Can you work these out from the model? Positions are in its coordinate system, mm. A direction names the side the tool comes from. Coordinates: 2 decimals unless noted, no trailing zeros. Loops run counter-clockwise (first coordinate to the right, second up) from the corner with the lowest first, then second, coordinate; pieces in that order, holes last.
Autodesk Inventor part; units mm, degrees
ref_plane "YZ Plane" through (0, 0, 0) normal (1, 0, 0) x (0, 1, 0)
ref_plane "XZ Plane" through (0, 0, 0) normal (0, 1, 0) x (-1, 0, 0)
ref_plane "XY Plane" through (0, 0, 0) normal (0, 0, 1) x (1, 0, 0)
sketch "Sketch1" plane through (0, 0, 0) normal (0, 1, 0) x (-1, 0, 0)
  line L0 (0, 0) -> (33, 0)
  line L1 (33, 0) -> (33, -12)
  line L2 (33, -12) -> (0, -12)
  line L3 (0, -12) -> (0, 0)
  circle A0 centre (26, -6) radius 3.25
  circle A1 centre (7, -6) radius 3.25
  dimension "d0" = 12
  dimension "d1" = 33
  dimension "d2" = 6.5
  dimension "d3" = 6.5
  dimension "d4" = 7
  dimension "d6" = 6
  dimension "d7" = 6
  dimension "d9" = 19
extrude "Extrusion1" add sketch "Sketch1" along normal mid plane 14
sketch "Sketch2" plane through (0, -7, -12) normal (0, 0, -1) x (-1, 0, 0)
  circle A0 centre (16.5, 7) radius 3.1
  line L0 (33, 14) -> (33, 0)
  line L1 (33, 0) -> (0, 0)
  point P0 (0, 7)
  dimension "d12" = 6.2
  dimension "d14" = 16.5
  dimension "d20" = 7
extrude "Extrusion2" cut sketch "Sketch2" against normal up to next
sketch "Sketch3" plane through (-33, -7, 0) normal (0, 0, 1) x (1, 0, 0)
  circle A0 centre (16.5, 7) radius 3.1
  line L0 (16.5, 13.0044) -> (21.7, 10.0022)
  line L1 (21.7, 10.0022) -> (21.7, 3.9978)
  line L2 (21.7, 3.9978) -> (16.5, 0.9956)
  line L3 (16.5, 0.9956) -> (11.3, 3.9978)
  line L4 (11.3, 3.9978) -> (11.3, 10.0022)
  line L5 (11.3, 10.0022) -> (16.5, 13.0044)
  line L6 (0, 14) -> (33, 14)
  line L7 (0, 14) -> (0, 0)
  point P0 (33, 7)
  dimension "d17" = 5.2
extrude "Extrusion3" cut sketch "Sketch3" against normal blind 5
properties part number "smallSprocketFixture" material "ABS Plastic"
Item 1: Suppose I cut it at C-C, the plane x = -26. Please give me the cut outline in (y, z).
Results are:
outline: (-7, -12) - (7, -12) - (7, -9.25) - (-7, -9.25) - close; (-7, -2.75) - (7, -2.75) - (7, 0) - (-7, 0) - close
Item 2: Suppose I cut it at B-B, the plane y = 0. Please give me the cut outline in (x, z).
Results are:
outline: (-33, -12) - (-19.6, -12) - (-19.6, -5) - (-21.7, -5) - (-21.7, 0) - (-33, 0) - close; (-13.4, -12) - (0, -12) - (0, 0) - (-11.3, 0) - (-11.3, -5) - (-13.4, -5) - close; hole circle Ø6.5 at (-26, -6); hole circle Ø6.5 at (-7, -6)
Item 3: I need wall thicknesses on line 1 along Z through (x, y) = (-26, 0); line 2 along Y through (x, z) = (-16.5, -7); line 3 along X through (y, z) = (0.25, -6.75). Which ranges of each line are inside material? Lowest first, please.
Results are:
line 1: z = -12 to -9.25, -2.75 to 0
line 2: y = -7 to -3.1, 3.1 to 7
line 3: x = -33 to -29.16, -22.84 to -19.59, -13.41 to -10.16, -3.84 to 0
Item 4: Suppose I cut it at D-D, the plane y = 4. Please give me the cut outline in (x, z).
Results are:
outline: (-33, -12) - (0, -12) - (0, 0) - (-13.03, 0) - (-13.03, -5) - (-19.97, -5) - (-19.97, 0) - (-33, 0) - close; hole circle Ø6.5 at (-26, -6); hole circle Ø6.5 at (-7, -6)
Item 5: On a 3-axis mill with a long thin cutter (end or side, diameter ignored), from which of +Z, -Z, +X, -X, +Y, -Y can I reach the whole of each face in a straight line? I mean faces 4 (the face through (-11.3, 0, -2)), 5 (the face through (-19.457, 0.931, -8.549)). Say none if no direction works.
Results are:
face 4: +Z
face 5: +Z, -Z
Item 6: Suppose I cut it at A-A, the plane z = -7.25. Please give me the cut outline in (x, y).
Results are:
outline: (-33, -7) - (-29, -7) - (-29, 7) - (-33, 7) - close; (-23, -7) - (-10, -7) - (-10, 7) - (-23, 7) - close; (-4, -7) - (0, -7) - (0, 7) - (-4, 7) - close; hole circle Ø6.2 at (-16.5, 0)
Item 7: I'm going to push a flat-ended pin straight in: P1, Ø2, axis at x = -27.5, y = -1, coming from the +Z side. Where does the tip first touch, or does it pass through?
Results are:
P1: stops at z = 0
Item 8: We'd pull the mould along Y, two halves only. Please class faces 1 (the face through (0, 0, -6)), 2 (the face through (-13.936, 4.524, -2.465)), 3 (the face through (-16, 7, -6)): +Y half, -Y half, draft (parallel to the pull), parting line (faces both ways), or undercut.
Results are:
face 1: draft
face 2: undercut
face 3: +Y half
